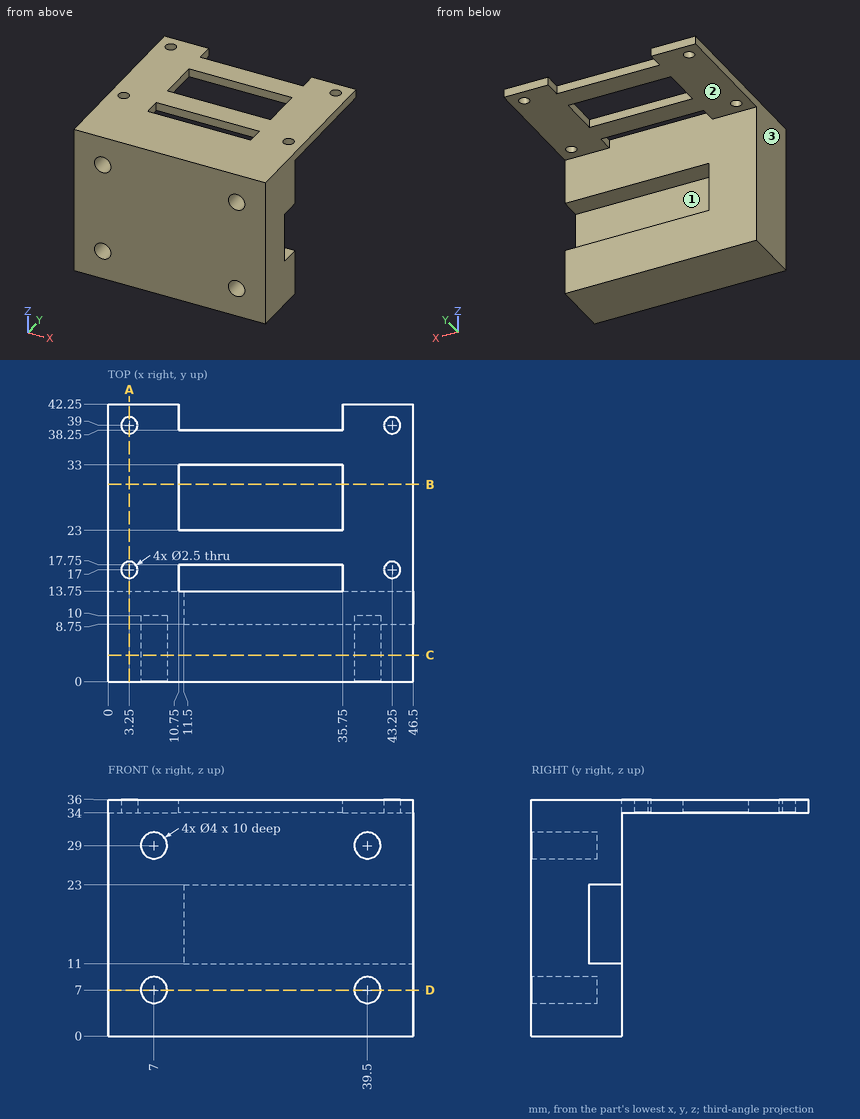
Geometry check sheet. Reference: drawing and pictorial views, mm from the part's lowest x, y, z. A direction names the side the tool comes from. Round coordinates to 2 decimals unless told otherwise and drop trailing zeros. Write each loop counter-clockwise with the first axis right and the second up, starting at its lowest first coordinate (ties: lowest second). Pieces come first, ordered by that corner, then holes. Notation, with made-up numbers: (75, 6) -> (108, 6) arc R21 ccw to (108, 25) -> close; hole circle Ø3 at (35, 10). An arc over 180 degrees is marked (long way). Answer as CSV lines item,"result". Start each with the question number.
1) Section check A-A on x = 3.25. Enter the section's corners in (y, z), and give its area (3 significant figures).
2) Material ranges on line 1 (X direction, y = 7, z = 7); line 2 (Y direction, x = 3.25, z = 35.6); line 3 (Z direction, x = 5.5, y = 7), recorded low to high. Write a range as from..to.
3) Section check D-D on z = 7. Enter the section's corners in (x, y).
4) Section check C-C on y = 4. Enter the section's corners in (x, z).
5) Section check B-B on y = 30. Enter the section's corners in (x, z), and give its area (3 significant figures).
6) Tool access check on the marked faces 1, 2 and 3. Record the directions out of +Z, -Z, +X, -X, +Y, -Y that give a thin tool (end or side, any length) a straight path to the whole face; none if there is none.
7) Go/stop test with flat-tipped pins: P1, Ø0.6, axis at x = 28.5, z = 35, coming from the +Y side; P2, Ø4.5, axis at x = 7, z = 7, coming from the +Y side; P3, Ø3, axis at x = 39.5, z = 29, coming from the -Y side. Record where each tip stops, or that it passes through.
Found:
1,outline,"(0, 0) -> (13.75, 0) -> (13.75, 34) -> (15.75, 34) -> (15.75, 36) -> (0, 36) -> close; (18.25, 34) -> (37.75, 34) -> (37.75, 36) -> (18.25, 36) -> close; (40.25, 34) -> (42.25, 34) -> (42.25, 36) -> (40.25, 36) -> close"
1,area,"542 mm^2"
2,line 1,"x = 0..5, 9..37.5, 41.5..46.5"
2,line 2,"y = 0..15.75, 18.25..37.75, 40.25..42.25"
2,line 3,"z = 0..5.68, 8.32..27.68, 30.32..36"
3,outline,"(0, 0) -> (5, 0) -> (5, 10) -> (9, 10) -> (9, 0) -> (37.5, 0) -> (37.5, 10) -> (41.5, 10) -> (41.5, 0) -> (46.5, 0) -> (46.5, 13.75) -> (0, 13.75) -> close"
4,outline,"(0, 0) -> (46.5, 0) -> (46.5, 36) -> (0, 36) -> close; hole circle Ø4 at (7, 7); hole circle Ø4 at (7, 29); hole circle Ø4 at (39.5, 7); hole circle Ø4 at (39.5, 29)"
5,outline,"(0, 34) -> (10.75, 34) -> (10.75, 36) -> (0, 36) -> close; (35.75, 34) -> (46.5, 34) -> (46.5, 36) -> (35.75, 36) -> close"
5,area,"43.0 mm^2"
6,face 1,"+X, +Y"
6,face 2,"-Z, +X, -X, +Y"
6,face 3,"+Z, -Z, -X, +Y, -Y"
7,P1,"stops at y = 38.25"
7,P2,"stops at y = 13.75"
7,P3,"stops at y = 10"
